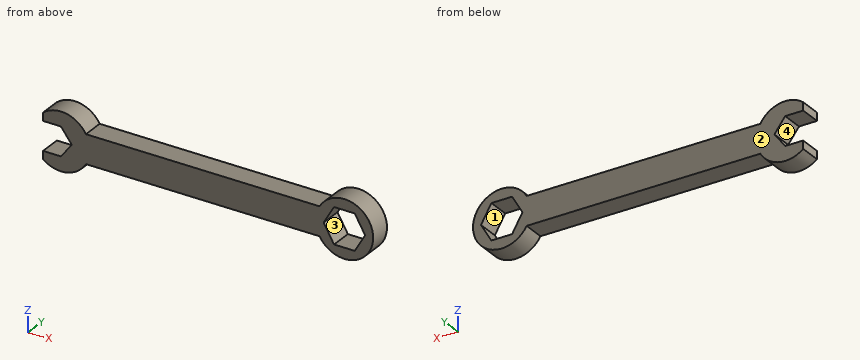
```python
from build123d import *

# Parameters (mm, degrees)
BOSS_EXTRUDE1_DEPTH = 7.62


with BuildPart() as part:
    # Sketch2 → Boss-Extrude1 (new body)
    with BuildSketch(Plane(origin=(0, 0, 0), x_dir=(1, 0, 0), z_dir=(0, 1, 0))):
        with BuildLine():
            Line((-41.275, 5.08), (41.275, 5.08))
            ThreePointArc((41.275, 5.08), (60.233818102, 0), (41.275, -5.08))
            Line((41.275, -5.08), (-41.275, -5.08))
            ThreePointArc((-41.275, -5.08), (-48.194606038, -9.984696391), (-56.423818102, -7.931147458))
            Line((-56.423818102, -7.931147458), (-56.423818102, -5.08))
            Line((-56.423818102, -5.08), (-50.073818102, -5.08))
            Line((-50.073818102, -5.08), (-46.263818102, 0))
            Line((-46.263818102, 0), (-50.073818102, 5.08))
            Line((-50.073818102, 5.08), (-56.423818102, 5.08))
            Line((-56.423818102, 5.08), (-56.423818102, 7.931147458))
            ThreePointArc((-56.423818102, 7.931147458), (-48.194606038, 9.984696391), (-41.275, 5.08))
        make_face()
        Polygon((53.739992312, -6.35), (57.406166521, 0), (53.739992312, 6.35), (46.407643893, 6.35), (42.741469684, 0), (46.407643893, -6.35), align=None, mode=Mode.SUBTRACT)
    extrude(amount=BOSS_EXTRUDE1_DEPTH)


solid = part.part
```
Design review of the part built by this model. Coordinates are the model's own, in mm. Face numbers are marked on the shaded views. Give positions to 0.01 mm unless a question says otherwise; leave off trailing zeros. Loops run counter-clockwise (first coordinate to the right, second up) from the corner with the lowest first, then second, coordinate; pieces in that order, holes last. Notation, with made-up numbers: (28.5, 66.25) -> (46.5, 66.25) arc R19 ccw to (46.5, 72.25) -> close; hole circle Ø1 at (72, 24.25). An arc over 180 degrees is marked (long way). One line per item, written item: value.
Q1. We need section D-D on z = -3.5. Give the boundary of the cut face in (x, y).
Numbers:
outline: (-48.89, 0) -> (44.76, 0) -> (44.76, 7.62) -> (-48.89, 7.62) -> close; (55.39, 0) -> (59.61, 0) -> (59.61, 7.62) -> (55.39, 7.62) -> close
Q2. We need section A-A on y = 3. Give the boundary of the cut face in (x, z) (3 decimals).
Numbers:
outline: (-56.424, -7.931) arc R10.16 ccw to (-41.275, -5.08) -> (41.275, -5.08) arc R10.16 ccw (long way) to (41.275, 5.08) -> (-41.275, 5.08) arc R10.16 ccw to (-56.424, 7.931) -> (-56.424, 5.08) -> (-50.074, 5.08) -> (-46.264, 0) -> (-50.074, -5.08) -> (-56.424, -5.08) -> close; hole (42.741, 0) -> (46.408, -6.35) -> (53.74, -6.35) -> (57.406, 0) -> (53.74, 6.35) -> (46.408, 6.35) -> close
Q3. For pin 1 Ø4 at (x, y) = (-15.5, 3.5) entering from -Z; pin 2 Ø3 at (x, y) = (-53, 4) entering from -Z; pin 3 Ø3 at (y, z) = (5.5, -1) entering from -X, all flat-tipped, find the tip position at first contact; note any pin that passes through.
Numbers:
pin 1: stops at z = -5.08
pin 2: stops at z = -10.06
pin 3: stops at x = -48.14
Q4. We need section B-B on z = 2.75. Give the boundary of the cut face in (x, y), and give its area (3 significant figures).
Numbers:
outline: (-48.33, 0) -> (44.33, 0) -> (44.33, 7.62) -> (-48.33, 7.62) -> close; (55.82, 0) -> (59.85, 0) -> (59.85, 7.62) -> (55.82, 7.62) -> close
area: 737 mm^2
Q5. We need section C-C on x = -31.5. Give the boundary of the cut face in (y, z).
Numbers:
outline: (0, -5.08) -> (7.62, -5.08) -> (7.62, 5.08) -> (0, 5.08) -> close
Q6. Draft analysis for pull direction X (two halves, no side actions). For the marked faces 1, 2, 3 and 4, state which applies: pulls with the +X half, pulls with the -X half, needs draft (parallel to the pull), parting line crosses it, or undercut.
Numbers:
face 1: undercut
face 2: needs draft
face 3: undercut
face 4: pulls with the -X half
Q7. For L1, parallel to X at y = 0.75, z = 5.25; L2, parallel to X at y = 5.75, z = -5.5; L3, parallel to Z at x = 4.5, y = 1.5, list the stretches that pass through material, from the lowest coordinate up.
Numbers:
L1: x = -56.42 to -41.38, 41.38 to 45.77, 54.38 to 58.77
L2: x = -56.42 to -41.53, 41.53 to 45.92, 54.23 to 58.62
L3: z = -5.08 to 5.08
